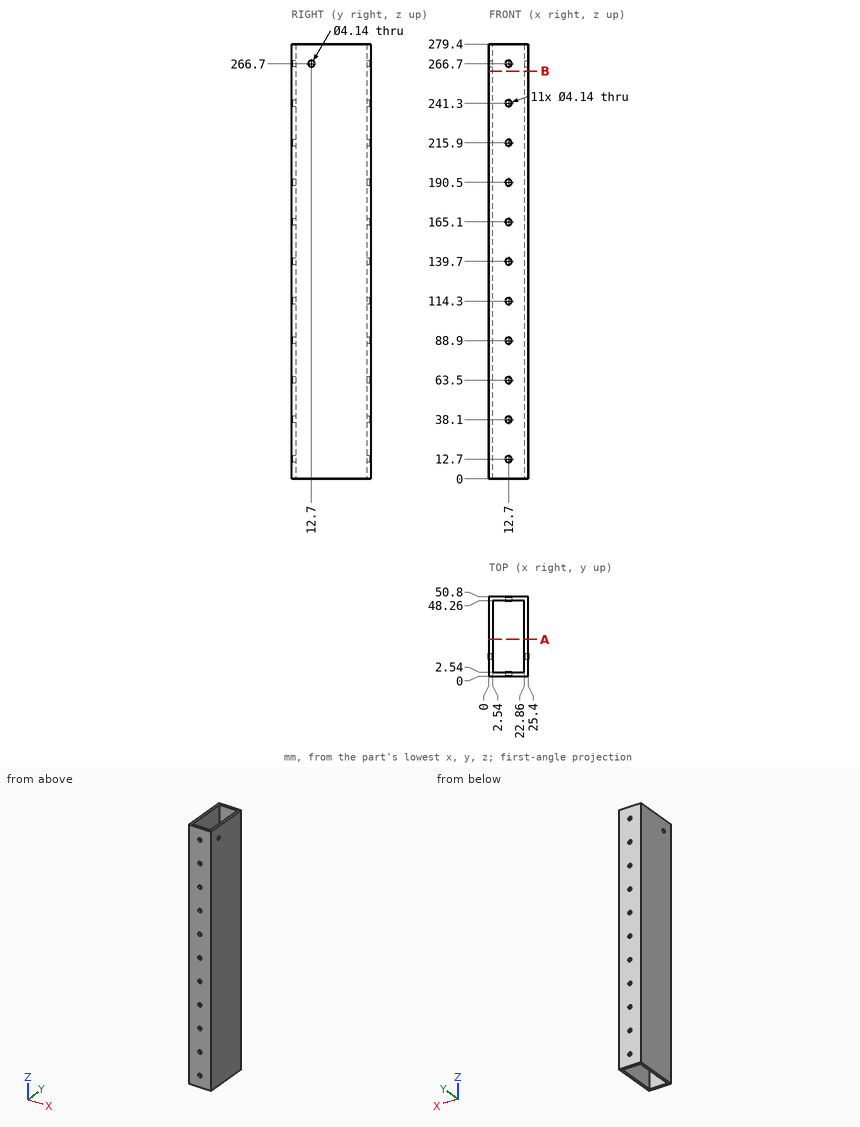
Print and shaded views of the part. All mm, measured from the part's lowest x, y and z. Coordinates: 2 decimals unless noted, no trailing zeros. Loops run counter-clockwise (first coordinate to the right, second up) from the corner with the lowest first, then second, coordinate; pieces in that order, holes last. Notation, with made-up numbers: (64, -26.75) - (115, -26.75) arc R9 cw to (115, -20.75) - close; hole circle Ø3 at (-35, 48). An arc over 180 degrees is marked (long way). Use one line per item in the form item = value. Start each with the question number.
1) Flat gauge pin, fed straight in: pin 1 (3.5 mm diameter, centred on x = 12.7, z = 241.3, fed in from -Y). Where does the tip first touch, or does it go through?
2) Drill centre lines: L1, parallel to X at y = 11.5, z = 44; L2, parallel to X at y = 49.1, z = 266.7; L3, parallel to Y at x = 21.5, z = 97.5. Where is each one in solid material? Low to high. Write a range as from..to.
3) Band-saw the part on A-A (y = 23.5). Give the cut face in (x, z).
4) Band-saw the part on B-B (z = 262). Give the cut face in (x, y), and give its area (3 significant figures).
Check values:
q1.pin_1 = through
q2.L1 = 0..2.54, 22.86..25.4
q2.L2 = 0..10.63, 14.77..25.4
q2.L3 = 0..2.54, 48.26..50.8
q3.outline = (0, 0) - (2.54, 0) - (2.54, 279.4) - (0, 279.4) - close; (22.86, 0) - (25.4, 0) - (25.4, 279.4) - (22.86, 279.4) - close
q4.outline = (0, 0) - (25.4, 0) - (25.4, 50.8) - (0, 50.8) - close; hole (2.54, 2.54) - (22.86, 2.54) - (22.86, 48.26) - (2.54, 48.26) - close
q4.area = 361 mm2
